Can you work these out from the drawing? Everything is in mm from the part's minimum corner. Give positions to 0.01 mm unless a question says otherwise; leave off trailing zeros. Loops run counter-clockwise (first coordinate to the right, second up) from the corner with the lowest first, then second, coordinate; pieces in that order, holes last. Notation, with made-up numbers: (39.5, 82.25) - (68.5, 82.25) arc R13 cw to (68.5, 107.25) - close; hole circle Ø9 at (60.25, -10.75). An arc over 180 degrees is marked (long way). Answer in a Markdown table with one row per item.
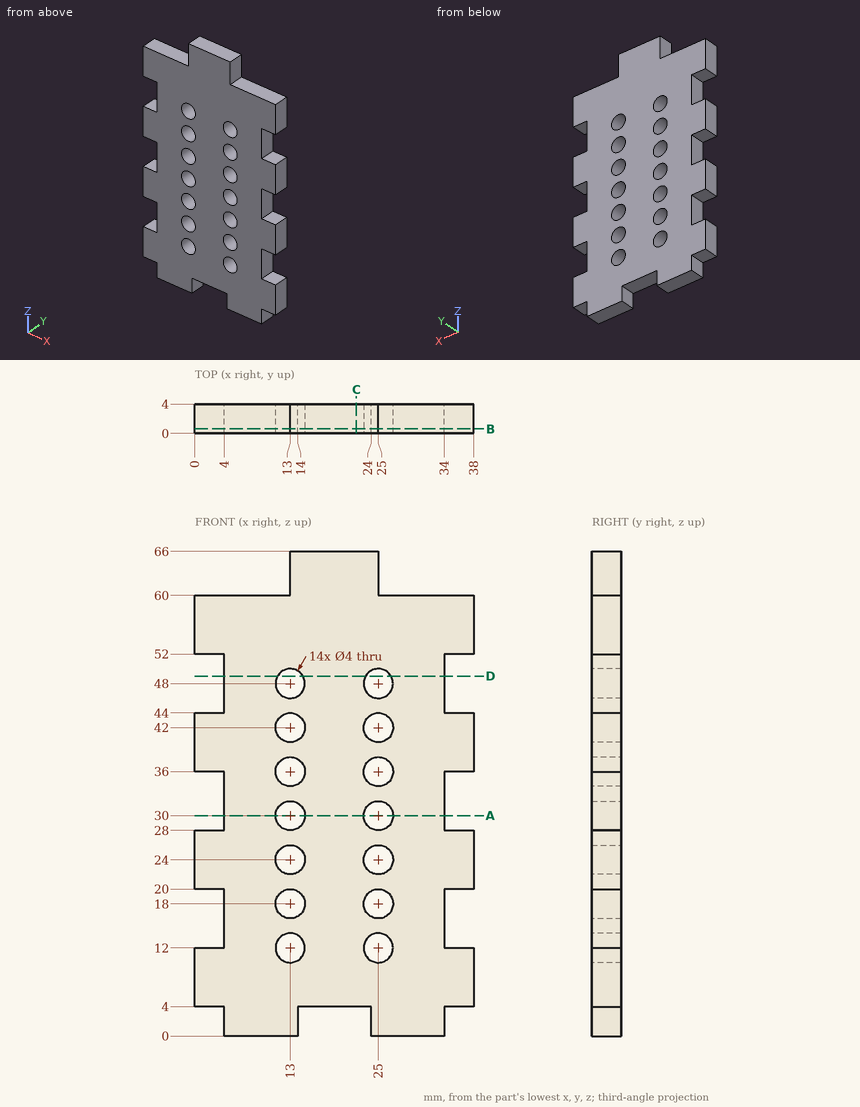
Q1. Imagine slicing it at B-B, the plane y = 0.6. Count the separate pieces of the cut face and the enclosed holes in it, and give its area (3 significant figures).
Checked values:
| item | result |
|---|---|
| separate pieces | 1 |
| enclosed holes | 14 |
| area | 1,910 mm² |
Q2. Imagine slicing it at C-C, the plane x = 22. Write out the boundary of the cut face in (y, z), and give its area (3 significant figures).
Checked values:
| item | result |
|---|---|
| outline | (0, 4) - (4, 4) - (4, 66) - (0, 66) - close |
| area | 248 mm² |
Q3. Imagine slicing it at D-D, the plane z = 49. Write out the boundary of the cut face in (x, y), and give its area (3 significant figures).
Checked values:
| item | result |
|---|---|
| outline | (4, 0) - (11.27, 0) - (11.27, 4) - (4, 4) - close; (14.73, 0) - (23.27, 0) - (23.27, 4) - (14.73, 4) - close; (26.73, 0) - (34, 0) - (34, 4) - (26.73, 4) - close |
| area | 92.3 mm² |
Q4. If I drill on line 1 (X direction, y = 1.1, z = 18); line 2 (X direction, y = 1, z = 42); line 3 (Z direction, x = 3, y = 2.4), over which ranges is the centre line in solid material (lowest first)? Write a range as [from, to].
Checked values:
| item | result |
|---|---|
| line 1 | x = [4, 11], [15, 23], [27, 34] |
| line 2 | x = [0, 11], [15, 23], [27, 38] |
| line 3 | z = [4, 12], [20, 28], [36, 44], [52, 60] |
Q5. Imagine slicing it at A-A, the plane z = 30. Write out the boundary of the cut face in (x, y), and give its area (3 significant figures).
Checked values:
| item | result |
|---|---|
| outline | (4, 0) - (11, 0) - (11, 4) - (4, 4) - close; (15, 0) - (23, 0) - (23, 4) - (15, 4) - close; (27, 0) - (34, 0) - (34, 4) - (27, 4) - close |
| area | 88.0 mm² |
Q6. For pin 1 (1.2 mm diameter, centred on x = 9.5, y = 3, fed in from +Z); pin 2 (2 mm diameter, centred on x = 36.5, y = 1.5, fed in from -Z); pin 3 (2 mm diameter, centred on y = 1.5, z = 14, fed in from +X), each with a flat end and sliding along its axis, tell me the tip position at first contact or that it passes through.
Checked values:
| item | result |
|---|---|
| pin 1 | stops at z = 60 |
| pin 2 | stops at z = 4 |
| pin 3 | stops at x = 34 |
